Design review of the part built by this model. Coordinates are the model's own, in mm. Give positions to 0.01 mm unless a question says otherwise; leave off trailing zeros. Write each loop counter-clockwise with the first axis right and the second up, starting at its lowest first coordinate (ties: lowest second). Pieces come first, ordered by that corner, then holes. Notation, with made-up numbers: (32.25, 25) -> (82.25, 25) arc R21 cw to (82.25, 52) -> close; hole circle Ø1 at (89.5, 11). An arc over 180 degrees is marked (long way). Answer as a JSON object with one key per item and string values.
```python
from build123d import *

# Parameters (mm, degrees)
SKETCH1_W                      = 457.2
SKETCH1_H                      = 88.9
BOSS_EXTRUDE1_DEPTH            = 88.9
SKETCH2_R                      = 22.225
CUT_EXTRUDE1_DEPTH             = 89.9
F_5_16_0_3125_DIAMETER_HOLE1_D = 7.9375
FILLET1_R                      = 4.7625


with BuildPart() as part:
    # Sketch1 → Boss-Extrude1 (new body)
    with BuildSketch(Plane.XY):
        with Locations((0, -527.543937925)):
            Rectangle(SKETCH1_W, SKETCH1_H)
    extrude(amount=-BOSS_EXTRUDE1_DEPTH)

    # Sketch2 → Cut-Extrude1 (cut, through all)
    with BuildSketch(Plane.XY):
        with Locations((164.309496882, -525.607187925)):
            Circle(SKETCH2_R)
        with Locations((-164.309496882, -525.607187925)):
            Circle(SKETCH2_R)
    extrude(amount=-CUT_EXTRUDE1_DEPTH, mode=Mode.SUBTRACT)

    # 5/16 (0.3125) Diameter Hole1 (through all)
    with Locations(Plane(origin=(0, -483.093937925, 0), x_dir=(1, 0, 0), z_dir=(0, 1, 0))):
        with Locations((-164.309496882, 25.4), (164.309496882, 25.4)):
            Hole(F_5_16_0_3125_DIAMETER_HOLE1_D / 2)

    # Fillet1
    fillet1_edges = [part.edges().sort_by_distance(p)[0] for p in [
        (0, -483.093937925, 0),
        (0, -571.993937925, -88.9),
        (0, -483.093937925, -88.9),
        (0, -571.993937925, 0),
    ]]
    fillet(fillet1_edges, radius=FILLET1_R)


solid = part.part
```
(1) The part is to be moulded in two halves that separate along X. For faces 1 (the flat face through (-3, -571.994, -44)), 2 (the cylindrical face through (-169.127, -547.304, -43.828)), 3 (the flat face through (-228.6, -528, -44)), say which applies: +X half, -X half, draft (parallel to the pull), parting line (faces both ways), or undercut.
Here are the results:
{"face 1": "draft", "face 2": "undercut", "face 3": "-X half"}
(2) We need section A-A, the plane z = -25.4. Give the number of separate pieces and of enclosed holes in the cut face, then the cut area to 3 significant figures.
Here are the results:
{"separate pieces": "3", "enclosed holes": "0", "area": "36,800 mm²"}
(3) We need section B-B, the plane x = -147. State the section outline as (y, z) points (1 decimal).
Here are the results:
{"outline": "(-572, -84.1) arc R4.8 ccw to (-567.2, -88.9) -> (-539.5, -88.9) -> (-539.5, 0) -> (-567.2, 0) arc R4.8 ccw to (-572, -4.8) -> close; (-511.7, -88.9) -> (-487.9, -88.9) arc R4.8 ccw to (-483.1, -84.1) -> (-483.1, -4.8) arc R4.8 ccw to (-487.9, 0) -> (-511.7, 0) -> close"}
(4) We need section C-C, the plane y = -534.5. State the section outline as (x, z) points.
Here are the results:
{"outline": "(-228.6, -88.9) -> (-184.68, -88.9) -> (-184.68, 0) -> (-228.6, 0) -> close; (-143.94, -88.9) -> (143.94, -88.9) -> (143.94, 0) -> (-143.94, 0) -> close; (184.68, -88.9) -> (228.6, -88.9) -> (228.6, 0) -> (184.68, 0) -> close"}
(5) For line 1 along X through (y, z) = (-492.75, -25.4); line 2 along X through (y, z) = (-561, -25); line 3 along Y through (x, z) = (-137, -4.5), list the stretches that pass through material, from the lowest coordinate up.
Here are the results:
{"line 1": "x = -228.6 to -168.28, -160.34 to 160.34, 168.28 to 228.6", "line 2": "x = -228.6 to -168.26, -160.36 to 160.36, 168.26 to 228.6", "line 3": "y = -571.99 to -483.1"}
(6) Clearance check with a flat-ended pin moving along its axis: pin 1 (7 mm diameter, centred on x = -164.31, z = -25.4, fed in from -Y). State where the tip first meets the part, or that it passes through.
Here are the results:
{"pin 1": "passes through"}
